Here's how the part is built. I have some questions about the finished solid (model axes, mm). Round coordinates to 2 decimals unless told otherwise and drop trailing zeros. Loops run counter-clockwise (first coordinate to the right, second up) from the corner with the lowest first, then second, coordinate; pieces in that order, holes last. Notation, with made-up numbers: M 33.5,53.5 L 65.5,53.5 A13 cw 65.5,66.5 Z; hole C -33.75,71.25 d9. An arc over 180 degrees is marked long. Use a Markdown table: item, result.
from build123d import *

# Parameters (mm, degrees)
SKETCH1_W           = 5.8
SKETCH1_H           = 7.9
BOSS_EXTRUDE1_DEPTH = 62
SKETCH2_R           = 1.6
CUT_EXTRUDE1_DEPTH  = 6.8
FILLET1_R           = 3


with BuildPart() as part:
    # Sketch1 → Boss-Extrude1 (new body)
    with BuildSketch(Plane.XY):
        Rectangle(SKETCH1_W, SKETCH1_H)
    extrude(amount=BOSS_EXTRUDE1_DEPTH)

    # Sketch2 → Cut-Extrude1 (cut, through all)
    with BuildSketch(Plane(origin=(2.9, 0, 0), x_dir=(0, 0, -1), z_dir=(1, 0, 0))):
        with Locations((-7.2, 0)):
            Circle(SKETCH2_R)
    extrude(amount=-CUT_EXTRUDE1_DEPTH, mode=Mode.SUBTRACT)

    # Fillet1
    fillet1_edges = [part.edges().sort_by_distance(p)[0] for p in [
        (0, 3.95, 62),
    ]]
    fillet(fillet1_edges, radius=FILLET1_R)


solid = part.part
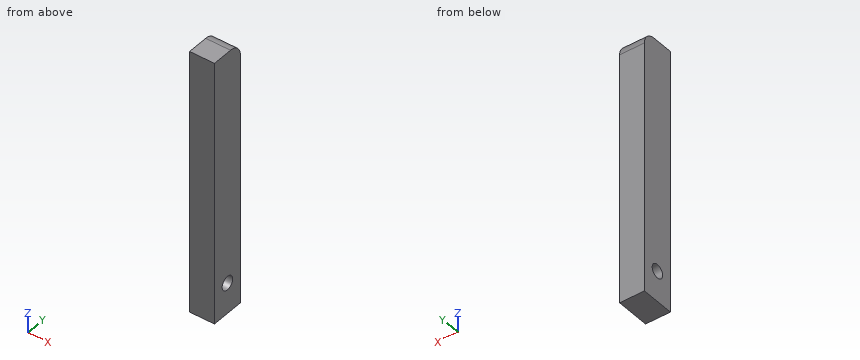
1. I need wall thicknesses on probe 1 along Y at (x, z) = (0.7, 7.2); probe 2 along Z at (x, y) = (-0.8, -1.25); probe 3 along Y at (x, z) = (2.45, 8.5). Which ranges of each line are inside material? Lowest first, please. Write a range as from..to.
Answer sheet:
| item | result |
|---|---|
| probe 1 | -3.95..-1.6, 1.6..3.95 |
| probe 2 | 0..6.2, 8.2..62 |
| probe 3 | -3.95..-0.93, 0.93..3.95 |
2. Imagine slicing it at B-B, the plane y = 0. Write out the boundary of the cut face in (x, z).
Answer sheet:
| item | result |
|---|---|
| outline | M -2.9,0 L 2.9,0 L 2.9,5.6 L -2.9,5.6 Z; M -2.9,8.8 L 2.9,8.8 L 2.9,62 L -2.9,62 Z |
3. Imagine slicing it at C-C, the plane x = 1.2. Write out the boundary of the cut face in (y, z), then the cut area to 3 significant figures.
Answer sheet:
| item | result |
|---|---|
| outline | M -3.95,0 L 3.95,0 L 3.95,59 A3 ccw 0.95,62 L -3.95,62 Z; hole C 0,7.2 d3.2 |
| area | 480 mm2 |
4. Imagine slicing it at A-A, the plane z = 7.2. Write out the boundary of the cut face in (x, y).
Answer sheet:
| item | result |
|---|---|
| outline | M -2.9,-3.95 L 2.9,-3.95 L 2.9,-1.6 L -2.9,-1.6 Z; M -2.9,1.6 L 2.9,1.6 L 2.9,3.95 L -2.9,3.95 Z |
